Geometry: final body of the model. Coordinates: model frame, mm. Give positions to 0.01 mm unless a question says otherwise; leave off trailing zeros. Loops run counter-clockwise (first coordinate to the right, second up) from the corner with the lowest first, then second, coordinate; pieces in that order, holes last. Notation, with made-up numbers: (-3.75, 37) - (40.25, 37) arc R22 cw to (40.25, 72) - close; hole circle Ø6 at (0, 8.5). An arc over 180 degrees is marked (long way). Answer in a Markdown table with one row per item.
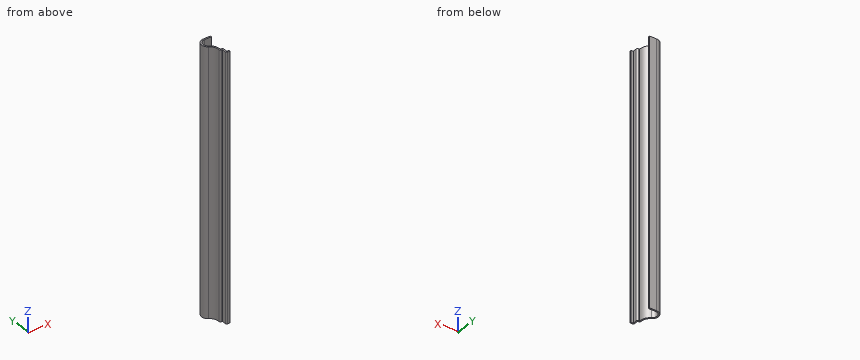
from build123d import *

# Parameters (mm, degrees)
EXTRUDE_THIN1_DEPTH = 238.125
FILLET1_R           = 1.27


with BuildPart() as part:
    # Sketch1 → Extrude-Thin1 (new body)
    with BuildSketch(Plane.XY):
        with BuildLine():
            Line((0, 0), (-3.175, 0))
            Line((-3.175, 0), (-3.175, 4.7625))
            Line((-3.175, 4.7625), (-5.55625, 4.7625))
            ThreePointArc((-5.55625, 4.7625), (-5.936639641, 9.724124929), (-9.196056015, 13.484260978))
            ThreePointArc((-9.196056015, 13.484260978), (-11.70659771, 19.732317421), (-6.35, 23.8125))
            Line((-6.35, 23.8125), (0, 23.8125))
            Line((0, 23.8125), (0, 22.5425))
            Line((0, 22.5425), (-6.35, 22.5425))
            ThreePointArc((-6.35, 22.5425), (-10.48223252, 19.394930582), (-8.545528926, 14.575001326))
            ThreePointArc((-8.545528926, 14.575001326), (-5.103452481, 10.935459111), (-4.076247664, 6.0325))
            Line((-4.076247664, 6.0325), (-1.905, 6.0325))
            Line((-1.905, 6.0325), (-1.905, 1.27))
            Line((-1.905, 1.27), (0, 1.27))
            Line((0, 1.27), (0, 0))
        make_face()
    extrude(amount=-EXTRUDE_THIN1_DEPTH)

    # Fillet1
    fillet1_edges = [part.edges().sort_by_distance(p)[0] for p in [
        (-1.905, 6.0325, -119.0625),
        (-3.175, 0, -119.0625),
        (-5.55625, 4.7625, -119.0625),
    ]]
    fillet(fillet1_edges, radius=FILLET1_R)


solid = part.part
Q1. Material intervals for line 1 along Y through (x, z) = (-4, -154); line 2 along Y through (x, z) = (-1.25, -34); line 3 along X through (y, z) = (14, -178.5), sorted ascending.
Check values:
| item | result |
|---|---|
| line 1 | 4.76 to 6.03, 22.54 to 23.81 |
| line 2 | 0 to 1.27, 22.54 to 23.81 |
| line 3 | -9.92 to -7.69 |
Q2. Cut plane B-B (y = 11.25). Output: boundary loops of the cut face in (x, z) (3 decimals), and give its area (3 significant figures).
Check values:
| item | result |
|---|---|
| outline | (-6.781, -238.125) - (-5.276, -238.125) - (-5.276, 0) - (-6.781, 0) - close |
| area | 358 mm² |
Q3. First-contact query: pin 1 (4 mm diameter, centred on y = 3.5, z = -97.5, fed in from -X); pin 2 (2 mm diameter, centred on y = 19, z = -183, fed in from +X); pin 3 (6 mm diameter, centred on x = -9.5, z = -44, fed in from -Y); pin 4 (1.5 mm diameter, centred on x = -6.5, y = 8.5, fed in from -Z). Flat tips, straight axial feed; report the tip coordinate or a pass-through.
Check values:
| item | result |
|---|---|
| pin 1 | x = -5.23 |
| pin 2 | x = -10.27 |
| pin 3 | y = 10.82 |
| pin 4 | through |
